```python
from build123d import *

# Parameters (mm, degrees)
F1_DEPTH = 46
F2_R     = 3
F3_DEPTH = 25
F4_R     = 4.5
F5_DEPTH = 25
F6_SIZE  = 2


with BuildPart() as f1:
    # F0 (on Right) → F1 (new body)
    with BuildSketch(Plane.YZ):
        Polygon((43, 0), (0, 0), (0, -52), (6, -52), (6, -6), (43, -6), align=None)
    extrude(amount=F1_DEPTH)

    # F2 (on Top) → F3 (cut)
    with BuildSketch(Plane.XY):
        with Locations((38.9, 15.5)):
            Circle(F2_R)
        with Locations((38.9, 34.5)):
            Circle(F2_R)
        with Locations((7.1, 15.5)):
            Circle(F2_R)
        with Locations((7.1, 34.5)):
            Circle(F2_R)
    extrude(amount=-F3_DEPTH, mode=Mode.SUBTRACT)

    # F4 (on face) → F5 (cut)
    with BuildSketch(Plane.XZ):
        with Locations((23, -19)):
            Circle(F4_R)
        with BuildLine():
            ThreePointArc((23, -37.5), (16.672627, -36.384313), (11.108429, -33.171822))
            ThreePointArc((11.108429, -33.171822), (4.768685, -33.726478), (5.323341, -40.066222))
            ThreePointArc((5.323341, -40.066222), (13.594446, -44.841547), (23, -46.5))
            ThreePointArc((23, -46.5), (27.5, -42), (23, -37.5))
        make_face()
    extrude(amount=-F5_DEPTH, mode=Mode.SUBTRACT)

    # F6
    f6_edges = [f1.edges().sort_by_distance(p)[0] for p in [
        (0, 43, -3),
        (46, 43, -3),
        (46, 3, -52),
        (0, 3, -52),
    ]]
    chamfer(f6_edges, length=F6_SIZE)


solid = f1.part
```
The model under review builds one solid part; all positions refer to its coordinate system, in mm. A direction names the side the tool comes from. Round coordinates to 2 decimals unless told otherwise and drop trailing zeros. Order: outer loops, then holes, each group sorted by start corner. A loop starts at its lowest first (then second) coordinate and runs counter-clockwise, first axis right, second up. Notation, with made-up numbers: (75.25, 71.25) -> (116.25, 71.25) arc R34 cw to (116.25, 107.25) -> close; hole circle Ø3 at (-33.75, 43). An arc over 180 degrees is marked (long way). One line per item, written item: value. Start each with the question number.
Q1. Take a section at B-B (x = 7.1). Write out the cut boundary in (y, z).
Q2. Take a section at C-C (y = 13.5). Write out the cut boundary in (x, z).
Q3. Wall thickness on line 1 (Z direction, x = 23, y = 1.6); line 2 (Y direction, x = 7, z = -4); line 3 (Y direction, x = 38, z = -2): over which ranges is each line inside the solid? List them lowest first.
Q4. Clearance check with flat-ended pins moving along their axes: pin 1 Ø8 at (x, y) = (13, 16) entering from +Z; pin 2 Ø4 at (x, y) = (28.5, 25) entering from -Z; pin 3 Ø10.5 at (x, z) = (23, -19) entering from +Y. State where each tip first meets the part, or that it passes through.
Q5. Machinability: for faces 4 (the face through (23, 24, -6)), 5 (the face through (27.5, 3, -42.1)), 6 (the face through (23, 43, -3)), which of the approach directions +Z, -Z, +X, -X, +Y, -Y give a long, thin tool a straight path to every point of the face, cutting with its end or side? Answer none if there is none.
Q6. Take a section at D-D (x = 29). Write out the cut boundary in (y, z).
Q7. Mouldability with a two-part tool opening along X and no side actions: class faces 1 (the face through (23, 6, -29)), 2 (the face through (16.758, 2.958, -36.415)), 3 (the face through (45, 42, -3)) as released by +X, released by -X, zero draft, split by the parting line, or undercut.
Q8. Take a section at A-A (z = -19). Write out the cut boundary in (x, y), and give its area (3 significant figures).
Reported:
1. outline: (0, -52) -> (6, -52) -> (6, -41.44) -> (0, -41.44) -> close; (0, -32.26) -> (6, -32.26) -> (6, -6) -> (12.5, -6) -> (12.5, 0) -> (0, 0) -> close; (18.5, -6) -> (31.5, -6) -> (31.5, 0) -> (18.5, 0) -> close; (37.5, -6) -> (43, -6) -> (43, 0) -> (37.5, 0) -> close
2. outline: (0, -6) -> (4.86, -6) -> (4.86, 0) -> (0, 0) -> close; (9.34, -6) -> (36.66, -6) -> (36.66, 0) -> (9.34, 0) -> close; (41.14, -6) -> (46, -6) -> (46, 0) -> (41.14, 0) -> close
3. line 1: z = -52 to -46.5, -37.5 to -23.5, -14.5 to 0
3. line 2: y = 0 to 12.5, 18.5 to 31.5, 37.5 to 43
3. line 3: y = 0 to 12.64, 18.36 to 31.64, 37.36 to 43
4. pin 1: stops at z = 0
4. pin 2: stops at z = -6
4. pin 3: stops at y = 6
5. face 4: -Z, +X, -X, +Y
5. face 5: +Y, -Y
5. face 6: +Z, -Z, +X, -X, +Y
6. outline: (0, -52) -> (6, -52) -> (6, -6) -> (43, -6) -> (43, 0) -> (0, 0) -> close
7. face 1: zero draft
7. face 2: undercut
7. face 3: released by +X
8. outline: (0, 0) -> (18.5, 0) -> (18.5, 6) -> (0, 6) -> close; (27.5, 0) -> (46, 0) -> (46, 6) -> (27.5, 6) -> close
8. area: 222 mm2
